from build123d import *

# Parameters (mm, degrees)
F0_W     = 22.633268
F0_H     = 12.269363
F1_DEPTH = 25
F2_R     = 22.308841
F3_DEPTH = 29.9
F5_SIZE  = 5
F6_SIZE  = 5


with BuildPart() as f1:
    # F0 (on Front) → F1 (new body)
    with BuildSketch(Plane.XZ):
        with Locations((11.316634, -6.134682)):
            Rectangle(F0_W, F0_H)
    extrude(amount=F1_DEPTH)

    # F5
    f5_edges = [f1.edges().sort_by_distance(p)[0] for p in [
        (22.633268, -12.5, 0),
    ]]
    chamfer(f5_edges, length=F5_SIZE)

    # F6
    f6_edges = [f1.edges().sort_by_distance(p)[0] for p in [
        (0, -12.5, 0),
    ]]
    chamfer(f6_edges, length=F6_SIZE)


with BuildPart() as f3:
    # F2 (on Top) → F3 (new body)
    with BuildSketch(Plane.XY):
        with Locations((-79.230487, 19.022213)):
            Circle(F2_R)
    extrude(amount=F3_DEPTH)


solid = f1.part
Design review of the part built by this model. Coordinates are the model's own, in mm. Coordinates: 2 decimals unless noted, no trailing zeros. Write each loop counter-clockwise with the first axis right and the second up, starting at its lowest first coordinate (ties: lowest second). Pieces come first, ordered by that corner, then holes. Notation, with made-up numbers: (85, 76.5) - (124, 76.5) arc R16 ccw to (124, 105.5) - close; hole circle Ø9 at (87.5, 15). An arc over 180 degrees is marked (long way). Use one line per item in the form item = value.
Q1. Consider section A-A (y = -11). Write out the cut boundary in (x, z).
Taken from the geometry:
outline = (0, -12.27) - (22.63, -12.27) - (22.63, -5) - (17.63, 0) - (5, 0) - (0, -5) - close
Q2. Consider section B-B (x = 4). Write out the cut boundary in (y, z).
Taken from the geometry:
outline = (-25, -12.27) - (0, -12.27) - (0, -1) - (-25, -1) - close
Q3. Consider section C-C (z = -4). Write out the cut boundary in (x, y).
Taken from the geometry:
outline = (1, -25) - (21.63, -25) - (21.63, 0) - (1, 0) - close
Q4. For probe 1 along X at (y, z) = (-11, -2.25); probe 2 along X at (y, z) = (-13.25, -2); probe 3 along Z at (x, y) = (21.75, -7.5), list the stretches that pass through material, from the lowest coordinate up.
Taken from the geometry:
probe_1 = 2.75 to 19.88
probe_2 = 3 to 19.63
probe_3 = -12.27 to -4.12
